Source: CAD feature listing. Evaluate the final solid. Frame: model axes, mm. A direction names the side the tool comes from. Give positions to 0.01 mm unless a question says otherwise; leave off trailing zeros. Order: outer loops, then holes, each group sorted by start corner. A loop starts at its lowest first (then second) coordinate and runs counter-clockwise, first axis right, second up.
from build123d import *

# Parameters (mm, degrees)
SKETCH1_W           = 85
SKETCH1_H           = 12
SKETCH1_R           = 1.5
BOSS_EXTRUDE1_DEPTH = 2
SKETCH1_3_W         = 85
SKETCH1_3_H         = 12
BOSS_EXTRUDE2_DEPTH = 4
SKETCH2_W           = 85
SKETCH2_H           = 3
BOSS_EXTRUDE3_DEPTH = 5.1
BOSS_EXTRUDE4_DEPTH = 1
BOSS_EXTRUDE5_DEPTH = 10
SKETCH5_W           = 32
SKETCH5_H           = 67
BOSS_EXTRUDE6_DEPTH = 2
SKETCH6_W           = 32
SKETCH6_H           = 2
BOSS_EXTRUDE7_DEPTH = 11
BOSS_EXTRUDE9_DEPTH = 65
SKETCH9_W           = 100.016978449
SKETCH9_H           = 38.136204689
CUT_EXTRUDE1_DEPTH  = 0.1
SKETCH10_R          = 1.5
CUT_EXTRUDE2_DEPTH  = 6.1


with BuildPart() as part:
    # Sketch1 → Boss-Extrude1 (new body)
    with BuildSketch(Plane(origin=(0, 0, 0), x_dir=(1, 0, 0), z_dir=(0, 1, 0))):
        with Locations((42.5, 6)):
            Rectangle(SKETCH1_W, SKETCH1_H)
        Polygon((81.732050808, 3), (83.464101615, 6), (81.732050808, 9), (78.267949192, 9), (76.535898385, 6), (78.267949192, 3), align=None, mode=Mode.SUBTRACT)
        Polygon((56.732050808, 3), (58.464101615, 6), (56.732050808, 9), (53.267949192, 9), (51.535898385, 6), (53.267949192, 3), align=None, mode=Mode.SUBTRACT)
        Polygon((31.732050808, 3), (33.464101615, 6), (31.732050808, 9), (28.267949192, 9), (26.535898385, 6), (28.267949192, 3), align=None, mode=Mode.SUBTRACT)
        Polygon((6.732050808, 3), (8.464101615, 6), (6.732050808, 9), (3.267949192, 9), (1.535898385, 6), (3.267949192, 3), align=None, mode=Mode.SUBTRACT)
        Polygon((3.267949192, 3), (6.732050808, 3), (8.464101615, 6), (6.732050808, 9), (3.267949192, 9), (1.535898385, 6), align=None)
        with Locations((5, 6)):
            Circle(SKETCH1_R, mode=Mode.SUBTRACT)
        Polygon((28.267949192, 3), (31.732050808, 3), (33.464101615, 6), (31.732050808, 9), (28.267949192, 9), (26.535898385, 6), align=None)
        with Locations((30, 6)):
            Circle(SKETCH1_R, mode=Mode.SUBTRACT)
        Polygon((53.267949192, 3), (56.732050808, 3), (58.464101615, 6), (56.732050808, 9), (53.267949192, 9), (51.535898385, 6), align=None)
        with Locations((55, 6)):
            Circle(SKETCH1_R, mode=Mode.SUBTRACT)
        Polygon((78.267949192, 3), (81.732050808, 3), (83.464101615, 6), (81.732050808, 9), (78.267949192, 9), (76.535898385, 6), align=None)
        with Locations((80, 6)):
            Circle(SKETCH1_R, mode=Mode.SUBTRACT)
    extrude(amount=BOSS_EXTRUDE1_DEPTH)

    # Sketch1<3> → Boss-Extrude2 (add)
    with BuildSketch(Plane(origin=(0, 0, 0), x_dir=(1, 0, 0), z_dir=(0, 1, 0))):
        with Locations((42.5, 6)):
            Rectangle(SKETCH1_3_W, SKETCH1_3_H)
        Polygon((81.732050808, 3), (83.464101615, 6), (81.732050808, 9), (78.267949192, 9), (76.535898385, 6), (78.267949192, 3), align=None, mode=Mode.SUBTRACT)
        Polygon((56.732050808, 3), (58.464101615, 6), (56.732050808, 9), (53.267949192, 9), (51.535898385, 6), (53.267949192, 3), align=None, mode=Mode.SUBTRACT)
        Polygon((31.732050808, 3), (33.464101615, 6), (31.732050808, 9), (28.267949192, 9), (26.535898385, 6), (28.267949192, 3), align=None, mode=Mode.SUBTRACT)
        Polygon((6.732050808, 3), (8.464101615, 6), (6.732050808, 9), (3.267949192, 9), (1.535898385, 6), (3.267949192, 3), align=None, mode=Mode.SUBTRACT)
    extrude(amount=BOSS_EXTRUDE2_DEPTH)

    # Sketch2 → Boss-Extrude3 (add)
    with BuildSketch(Plane(origin=(0, 4, 0), x_dir=(1, 0, 0), z_dir=(0, 1, 0))):
        with Locations((42.5, 13.5)):
            Rectangle(SKETCH2_W, SKETCH2_H)
    extrude(amount=-BOSS_EXTRUDE3_DEPTH)

    # Sketch3 → Boss-Extrude4 (add)
    with BuildSketch(Plane.XZ.offset(1.1)):
        Polygon((85, -12), (0, -12), (0, -144.5), (55, -144.5), (55, -79.5), (85, -79.5), align=None)
    extrude(amount=-BOSS_EXTRUDE4_DEPTH)

    # Sketch4 → Boss-Extrude5 (add)
    with BuildSketch(Plane.XZ.offset(1.1)):
        Polygon((85, -79.5), (85, -77.5), (53, -77.5), (53, -144.5), (55, -144.5), (55, -79.5), align=None)
    extrude(amount=BOSS_EXTRUDE5_DEPTH)

    # Sketch5 → Boss-Extrude6 (add)
    with BuildSketch(Plane.XZ.offset(11.1)):
        with Locations((69, -111)):
            Rectangle(SKETCH5_W, SKETCH5_H)
    extrude(amount=-BOSS_EXTRUDE6_DEPTH)

    # Sketch6 → Boss-Extrude7 (add)
    with BuildSketch(Plane.XZ.offset(11.1)):
        with Locations((69, -143.5)):
            Rectangle(SKETCH6_W, SKETCH6_H)
    extrude(amount=-BOSS_EXTRUDE7_DEPTH)

    # Sketch8 → Boss-Extrude9 (add)
    with BuildSketch(Plane(origin=(0, 0, -144.5), x_dir=(-1, 0, 0), z_dir=(0, 0, -1))):
        Polygon((-55.130583843, -11.1), (-55.130583843, -0.1), (-69, -11.1), align=None)
    extrude(amount=-BOSS_EXTRUDE9_DEPTH)

    # Sketch9 → Cut-Extrude1 (cut)
    with BuildSketch(Plane(origin=(0, 0, -144.5), x_dir=(-1, 0, 0), z_dir=(0, 0, -1))):
        with Locations((-50.008489225, -19.168102345)):
            Rectangle(SKETCH9_W, SKETCH9_H)
    extrude(amount=-CUT_EXTRUDE1_DEPTH, mode=Mode.SUBTRACT)

    # Sketch10 → Cut-Extrude2 (cut, through all)
    with BuildSketch(Plane.XZ.offset(1.1)):
        with Locations((15, -121.9)):
            Circle(SKETCH10_R)
        with Locations((40, -121.9)):
            Circle(SKETCH10_R)
    extrude(amount=-CUT_EXTRUDE2_DEPTH, mode=Mode.SUBTRACT)


solid = part.part
(1) Section A-A, the plane x = 30. Return loops of the section in (y, z).
(2) Line query: line 1 along X through (y, z) = (0.45, -6); line 2 along Z through (x, y) = (80, 1.2); line 3 along Z through (x, y) = (15, -0.4). Output: solid intervals per line, ascending.
(3) Pin query (flat end, axial travel): pin 1 Ø2 at (x, z) = (20, -21) entering from -Y; pin 2 Ø1.2 at (x, y) = (34.5, -1) entering from +Z; pin 3 Ø1.8 at (x, z) = (54.5, -7.5) entering from +Y. Return the tip coordinate at first contact, or that it passes through.
(4) Access query for faces 4 (the flat face through (53, -6, -110)), 5 (the flat face through (0, -0.4, -55.8)), 6 (the flat face through (60.73, -4.54, -111.44)), 7 (the flat face through (42, 0, -6)), 8 (the flat face through (56.5, 2, -6.7)). Directions: +Z, -Z, +X, -X, +Y, -Y. A direction counts if a zero-diameter tool reaches every point of the face in a straight line with its end or side. Return the directions, or none.
(5) Section D-D, the plane x = 40. Return loops of the section in (y, z), plus the area to 3 significant figures.
(6) Draft query along Z for faces 1 (the flat face through (42, -0.1, -79)), 2 (the cylindrical face through (28.5, 0.99, -6.07)), 3 (the flat face through (69, -6, -77.5)). Return one class per face: +Z half, -Z half, draft (parallel to the pull), parting line (faces both ways), or undercut.
(7) Section C-C, the plane x = 18.5. Return loops of the section in (y, z).
(8) Section B-B, the plane y = -6.25. Return loops of the section in (x, z).
Checks:
1. outline: (-1.1, -144.4) - (-0.1, -144.4) - (-0.1, -15) - (4, -15) - (4, -9) - (2, -9) - (2, -7.5) - (0, -7.5) - (0, -12) - (-1.1, -12) - close; (0, -4.5) - (2, -4.5) - (2, -3) - (4, -3) - (4, 0) - (0, 0) - close
2. line 1: x = 0 to 3.5, 6.5 to 28.5, 31.5 to 53.5, 56.5 to 78.5, 81.5 to 85
2. line 2: z = -15 to -7.5, -4.5 to 0
2. line 3: z = -144.4 to -123.4, -120.4 to -12
3. pin 1: stops at y = -1.1
3. pin 2: stops at z = -12
3. pin 3: stops at y = 2
4. face 4: +Z, -Z, -X, -Y
4. face 5: +Z, -Z, -X, +Y, -Y
4. face 6: +X, +Y
4. face 7: +Z, +X, -X, -Y
4. face 8: +Y
5. outline: (-1.1, -144.4) - (-0.1, -144.4) - (-0.1, -123.4) - (-1.1, -123.4) - close; (-1.1, -120.4) - (-0.1, -120.4) - (-0.1, -15) - (4, -15) - (4, 0) - (0, 0) - (0, -12) - (-1.1, -12) - close
5. area: 190 mm2
6. face 1: draft
6. face 2: undercut
6. face 3: +Z half
7. outline: (-1.1, -144.4) - (-0.1, -144.4) - (-0.1, -15) - (4, -15) - (4, 0) - (0, 0) - (0, -12) - (-1.1, -12) - close
8. outline: (53, -144.4) - (85, -144.4) - (85, -142.5) - (62.88, -142.5) - (62.88, -79.5) - (85, -79.5) - (85, -77.5) - (53, -77.5) - close; hole (55, -142.5) - (55.13, -142.5) - (55.13, -79.5) - (55, -79.5) - close
